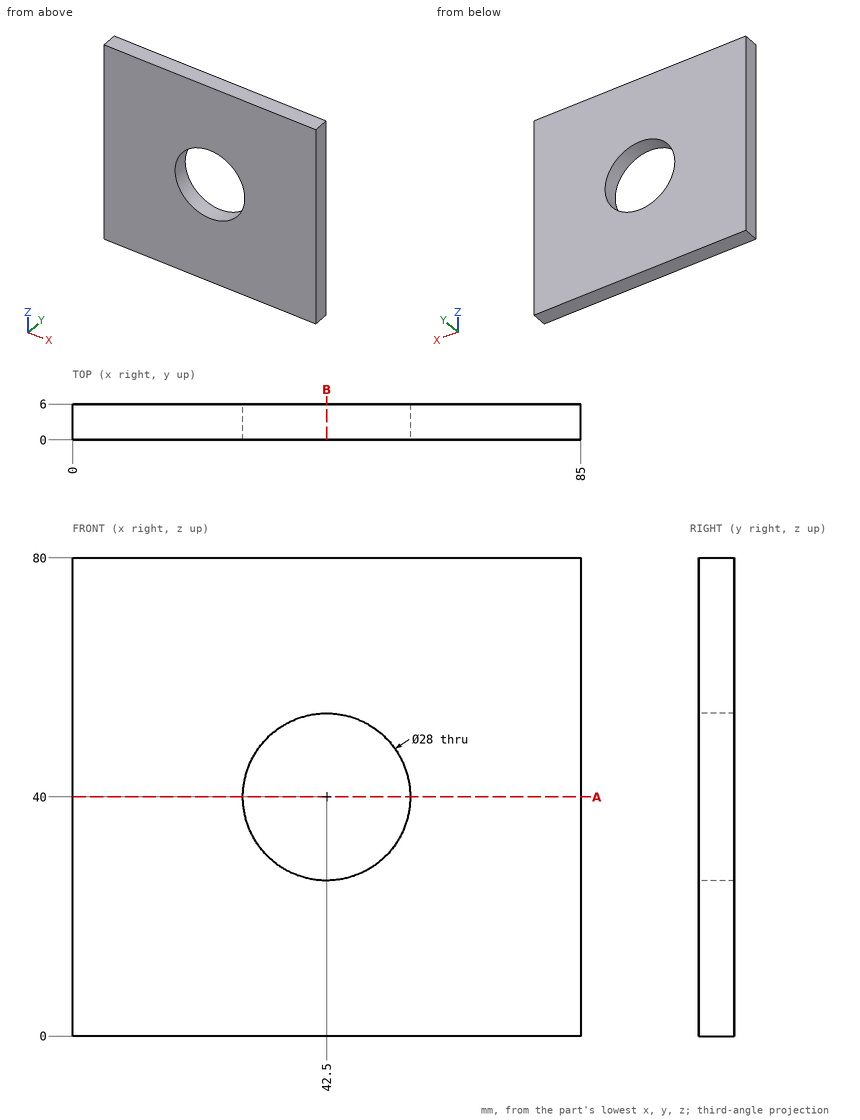
Verification items for this drawing (mm, ordinates from the low corner). Give positions to 0.01 mm unless a question says otherwise; leave off trailing zeros. Order: outer loops, then holes, each group sorted by start corner. A loop starts at its lowest first (then second) coordinate and runs counter-clockwise, first axis right, second up.
1) Cross-section at B-B (x = 42.5). Record the boundary of the cut face in (y, z).
Results are:
outline: (0, 0) - (6, 0) - (6, 26) - (0, 26) - close; (0, 54) - (6, 54) - (6, 80) - (0, 80) - close
2) Cross-section at A-A (z = 40). Record the boundary of the cut face in (x, y), then the cut area to 3 significant figures.
Results are:
outline: (0, 0) - (28.5, 0) - (28.5, 6) - (0, 6) - close; (56.5, 0) - (85, 0) - (85, 6) - (56.5, 6) - close
area: 342 mm2
3) Material ranges on probe 1 along Z at (x, y) = (42.5, 1.3); probe 2 along Z at (x, y) = (32, 3.55); probe 3 along X at (y, z) = (2.9, 46), recorded low to high.
Results are:
probe 1: z = 0 to 26, 54 to 80
probe 2: z = 0 to 30.74, 49.26 to 80
probe 3: x = 0 to 29.85, 55.15 to 85
